Read the model definition and answer for the solid it produces. Units are mm, in the model's axes. A direction names the side the tool comes from. Coordinates: 2 decimals unless noted, no trailing zeros. Write each loop counter-clockwise with the first axis right and the second up, starting at its lowest first coordinate (ties: lowest second). Pieces come first, ordered by that corner, then holes.
(1) Determine the mould class of faces 6 (the flat face through (0, 10, 9)), 7 (the flat face through (0, -6, 7)), 8 (the cylindrical face through (0, 0, 2)), 9 (the cylindrical face through (-7.87, 3.34, 8.97)) for opening direction Y: pulls with the +Y half, pulls with the -Y half, needs draft (parallel to the pull), parting line crosses it, or undercut.
(2) The part is cut by section B-B, the plane z = 8.25. Determine the outline of the cut face in (x, y).
(3) Which of the six approach directions +Z, -Z, +X, -X, +Y, -Y give full straight-line access (tool end or side, diameter ignored) to faces 1 (the flat face through (0, 2, 4)), 2 (the flat face through (0, -2, 3)), 3 (the cylindrical face through (-11.933, 1.402, 4.229)), 4 (the cylindrical face through (-7.87, -6.66, 8.97)), 5 (the cylindrical face through (11.902, -1.433, 4.327))?
(4) The part is cut by section A-A, the plane x = -7.5. Determine the outline of the cut face in (y, z).
(5) The part is cut by section C-C, the plane y = 5. Determine the outline of the cut face in (x, z).
(6) Straight lines are drawn through the part: line 1 along X through (y, z) = (5, 8.05); line 2 along Y through (x, z) = (-7.5, 9.15); line 3 along Z through (x, y) = (-9.75, -4.25). For each, find the intervals that lie inside material, in ascending order.
(7) Given pin 1 (3 mm diameter, centred on x = 1, y = 4.5, fed in from -Z); pin 2 (5.5 mm diameter, centred on x = -1.5, z = 3.5, fed in from -Y); pin 3 (4 mm diameter, centred on x = 7.5, y = -5, fed in from +Z), each flat-ended and moving along its own axis, determine where each tip first touches the part or whether it passes through.
```python
from build123d import *

# Parameters (mm, degrees)
PAD_DEPTH         = 12.5
SKETCH001_R       = 1.7
POCKET_DEPTH      = 0.001
POCKET_DEPTH_BACK = -11.001
FILLET_R          = 3
FILLET001_R       = 1.99


with BuildPart() as part:
    # Sketch → Pad (new body, symmetric)
    with BuildSketch(Plane.YZ):
        with BuildLine():
            Line((-2, 0), (-2, 7))
            Line((-2, 7), (-10, 7))
            Line((-10, 7), (-10, 11))
            Line((-10, 11), (10, 11))
            Line((10, 11), (10, 7))
            Line((10, 7), (2, 7))
            Line((2, 7), (2, 0))
            ThreePointArc((2, 0), (0, 2), (-2, 0))
        make_face()
    extrude(amount=PAD_DEPTH, both=True)

    # Sketch001 → Pocket (cut, two sides)
    with BuildSketch(Plane.XY) as pocket_sk:
        with Locations((-7.5, 5)):
            Circle(SKETCH001_R)
        with Locations((-7.5, -5)):
            Circle(SKETCH001_R)
        with Locations((7.5, 5)):
            Circle(SKETCH001_R)
        with Locations((7.5, -5)):
            Circle(SKETCH001_R)
    extrude(amount=-POCKET_DEPTH, mode=Mode.SUBTRACT)
    extrude(pocket_sk.sketch, amount=-POCKET_DEPTH_BACK, mode=Mode.SUBTRACT)

    # Fillet
    fillet_edges = [part.edges().sort_by_distance(p)[0] for p in [
        (12.5, 10, 9),
        (12.5, -10, 9),
        (-12.5, -10, 9),
        (-12.5, 10, 9),
    ]]
    fillet(fillet_edges, radius=FILLET_R)

    # Fillet001
    fillet001_edges = [part.edges().sort_by_distance(p)[0] for p in [
        (-12.5, -2, 3.5),
        (-12.5, 2, 3.5),
        (12.5, -2, 3.5),
        (12.5, 2, 3.5),
    ]]
    fillet(fillet001_edges, radius=FILLET001_R)


solid = part.part
```
Computed:
1. face 6: pulls with the +Y half
1. face 7: needs draft
1. face 8: undercut
1. face 9: undercut
2. outline: (-12.5, -7) arc R3 ccw to (-9.5, -10) - (9.5, -10) arc R3 ccw to (12.5, -7) - (12.5, 7) arc R3 ccw to (9.5, 10) - (-9.5, 10) arc R3 ccw to (-12.5, 7) - close; hole circle Ø3.4 at (-7.5, -5); hole circle Ø3.4 at (-7.5, 5); hole circle Ø3.4 at (7.5, -5); hole circle Ø3.4 at (7.5, 5)
3. face 1: -Z, +X, -X, +Y
3. face 2: -Z, +X, -X, -Y
3. face 3: -Z, -X, +Y
3. face 4: +Z, -Z
3. face 5: -Z, +X, -Y
4. outline: (-10, 7) - (-6.7, 7) - (-6.7, 11) - (-10, 11) - close; (-3.3, 7) - (-2, 7) - (-2, 0) arc R2 cw to (2, 0) - (2, 7) - (3.3, 7) - (3.3, 11) - (-3.3, 11) - close; (6.7, 7) - (10, 7) - (10, 11) - (6.7, 11) - close
5. outline: (-12.5, 7) - (-9.2, 7) - (-9.2, 11) - (-12.5, 11) - close; (-5.8, 7) - (5.8, 7) - (5.8, 11) - (-5.8, 11) - close; (9.2, 7) - (12.5, 7) - (12.5, 11) - (9.2, 11) - close
6. line 1: x = -12.5 to -9.2, -5.8 to 5.8, 9.2 to 12.5
6. line 2: y = -10 to -6.7, -3.3 to 3.3, 6.7 to 10
6. line 3: z = 7 to 11
7. pin 1: stops at z = 7
7. pin 2: stops at y = -2
7. pin 3: stops at z = 11
